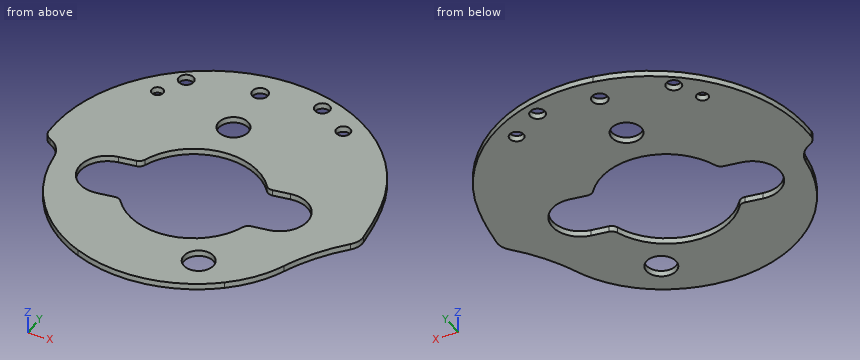
from build123d import *

# Parameters (mm, degrees)
BOSS_EXTRUDE1_DEPTH = 1.6
SKETCH2_R           = 4
SKETCH2_R_2         = 2
SKETCH2_R_3         = 1.551240763
SKETCH2_R_4         = 2.096920304
SKETCH2_R_5         = 1.874340877
CUT_EXTRUDE1_DEPTH  = 1.6
FILLET1_R           = 3
FILLET2_R           = 5


with BuildPart() as part:
    # Model → Boss-Extrude1 (new body)
    with BuildSketch(Plane.XY):
        with BuildLine():
            add(Edge.make_bspline(
                [(44.0581, -11.3354), (38.4033, 9.8661), (17.3587, 23.1222), (-4.2058, 19.0663)],
                knots=[0, 0, 0, 0, 0.333333333, 0.333333333, 0.333333333, 0.333333333], degree=3))
            add(Edge.make_bspline(
                [(-4.2058, 19.0663), (-25.7703, 15.0105), (-40.5609, -4.9853), (-38.1268, -26.7925)],
                knots=[0.333333333, 0.333333333, 0.333333333, 0.333333333, 1, 1, 1, 1], degree=3))
            add(Edge.make_bspline(
                [(-32.2525, -32.9684), (-32.6837, -29.8631), (-35.047, -27.3785), (-38.1268, -26.7925)],
                knots=[0, 0, 0, 0, 1, 1, 1, 1], degree=3))
            add(Edge.make_bspline(
                [(-32.2525, -32.9684), (-30.442, -46.0069), (-21.6996, -57.0365), (-9.4187, -61.7758)],
                knots=[0, 0, 0, 0, 0.333333333, 0.333333333, 0.333333333, 0.333333333], degree=3))
            add(Edge.make_bspline(
                [(-9.4187, -61.7758), (2.8622, -66.5152), (16.7476, -64.218), (26.8478, -55.776)],
                knots=[0.333333333, 0.333333333, 0.333333333, 0.333333333, 1, 1, 1, 1], degree=3))
            add(Edge.make_bspline(
                [(26.8478, -55.776), (30.8425, -52.4371), (33.9303, -48.1443), (35.8253, -43.295)],
                knots=[0, 0, 0, 0, 1, 1, 1, 1], degree=3))
            add(Edge.make_bspline(
                [(46.7562, -26.4745), (42.0043, -31.2778), (38.2846, -37.0019), (35.8253, -43.295)],
                knots=[0, 0, 0, 0, 1, 1, 1, 1], degree=3))
            add(Edge.make_bspline(
                [(46.7562, -26.4745), (46.284, -21.3612), (45.3815, -16.2969), (44.0581, -11.3354)],
                knots=[0, 0, 0, 0, 1, 1, 1, 1], degree=3))
        make_face()
    extrude(amount=BOSS_EXTRUDE1_DEPTH)

    # Sketch2 → Cut-Extrude1 (cut)
    with BuildSketch(Plane.XY.offset(1.6)):
        with Locations((17.3961, -51.3806)):
            Circle(SKETCH2_R)
        with Locations((-1.2327, -2.0433)):
            Circle(SKETCH2_R)
        with Locations((-20.0573, 8.5758)):
            Circle(SKETCH2_R_2)
        with Locations((13.2993, 14.7207)):
            Circle(SKETCH2_R_2)
        with Locations((-23.737719808, 1.389021653)):
            Circle(SKETCH2_R_3)
        with Locations((-2.328258131, 12.576412767)):
            Circle(SKETCH2_R_4)
        with Locations((21.984264555, 9.420615455)):
            Circle(SKETCH2_R_5)
        with BuildLine():
            Line((-19.056077425, -25.461514873), (-14.652380487, -24.690905022))
            ThreePointArc((-14.652380487, -24.690905022), (-13.702265565, -24.245091556), (-13.108712216, -23.379549857))
            ThreePointArc((-13.108712216, -23.379549857), (0.398385158, -11.905192157), (16.999343908, -18.110893783))
            ThreePointArc((16.999343908, -18.110893783), (17.85155014, -18.723439741), (18.896596337, -18.820116826))
            Line((18.896596337, -18.820116826), (23.300293275, -18.049506976))
            ThreePointArc((23.300293275, -18.049506976), (31.980824426, -24.144453977), (25.885877425, -32.824985127))
            Line((25.885877425, -32.824985127), (21.482180487, -33.595594978))
            ThreePointArc((21.482180487, -33.595594978), (20.532065565, -34.041408444), (19.938512216, -34.906950143))
            ThreePointArc((19.938512216, -34.906950143), (6.431414842, -46.381307843), (-10.169543908, -40.175606217))
            ThreePointArc((-10.169543908, -40.175606217), (-11.02175014, -39.563060259), (-12.066796337, -39.466383174))
            Line((-12.066796337, -39.466383174), (-16.470493275, -40.236993024))
            ThreePointArc((-16.470493275, -40.236993024), (-25.151024426, -34.142046023), (-19.056077425, -25.461514873))
        make_face()
    extrude(amount=-CUT_EXTRUDE1_DEPTH, mode=Mode.SUBTRACT)

    # Fillet1
    fillet1_edges = [part.edges().sort_by_distance(p)[0] for p in [
        (-38.1268, -26.7925, 0.8),
    ]]
    fillet(fillet1_edges, radius=FILLET1_R)

    # Fillet2
    fillet2_edges = [part.edges().sort_by_distance(p)[0] for p in [
        (46.7562, -26.4745, 0.8),
    ]]
    fillet(fillet2_edges, radius=FILLET2_R)


solid = part.part
Model file for the job. Use its own axes, mm. Give positions to 0.01 mm unless a question says otherwise; leave off trailing zeros. Return JSON: item names as keys, results as strings.
1) Cut at A-A, the plane z = 0.85. Count the separate pieces of the cut face and the enclosed holes in it, plus the area to 3 significant figures.
Geometry says:
{"separate pieces": "1", "enclosed holes": "8", "area": "3,900 mm²"}
2) Probe line 1 (Y direction, x = 16, z = 1.2); line 2 (X direction, y = 14, z = 1.55); line 3 (Y direction, x = -8.5, z = 0.3). List the from-to ranges inside material, lowest first. Write a range as from..to.
Geometry says:
{"line 1": "-62.02..-55.13, -47.63..-41.3, -16.98..17.9", "line 2": "-17.73..-3.87, -0.79..11.43, 15.16..24.8", "line 3": "-62.12..-41.96, -16.33..18.02"}
3) Flat gauge pin, fed straight in: P1, Ø7, axis at x = -1.23, y = -2.04, coming from the +Z side. Where does the tip first touch, or does it go through?
Geometry says:
{"P1": "through"}
